Check sheet for the modelled part. Datum: model origin and axes. Units: mm. A direction names the side the tool comes from. Round coordinates to 2 decimals unless told otherwise and drop trailing zeros. Order: outer loops, then holes, each group sorted by start corner. A loop starts at its lowest first (then second) coordinate and runs counter-clockwise, first axis right, second up. Notation, with made-up numbers: (-35.75, 15.5) -> (-24.75, 15.5) arc R15 cw to (-24.75, 38.5) -> close; hole circle Ø2 at (14.5, 67). An arc over 180 degrees is marked (long way). Answer in a Markdown table with one row per item. Add a question column.
1. Sectioned sample at C-C, the plane y = 439. Record the boundary of the cut face in (x, z), then the cut area to 3 significant figures.
2. Sectioned sample at B-B, the plane y = 164. Record the boundary of the cut face in (x, z).
3. Access from +Z, -Z, +X, -X, +Y, -Y to the whole of each face (thin tool, end or side, straight path). Record for faces 1 (the flat face through (370, 93, 0)), 2 (the flat face through (0, 507, -20)), 3 (the flat face through (379, 156, -23.207)).
4. Sectioned sample at D-D, the plane x = 431. Count the separate pieces of the cut face and the enclosed holes in it, then the cut area to 3 significant figures.
5. Material ranges on L1, parallel to Y at x = 413, z = -40; L2, parallel to Y at x = 228, z = -47; L3, parallel to X at y = 914.5, z = -28.5, recorded low to high. Write a range as from..to.
6. Draft check along Y on faces 4 (the flat face through (370, 1000, -20)), 5 (the flat face through (50, 93, -30)), 6 (the flat face through (750, 507, -20)). Enter one of: +Y half, -Y half, draft (parallel to the pull), parting line (faces both ways), or undercut.
7. Depth check by flat-ended pin: P1, Ø4, axis at x = 593, z = 8.5, coming from the -Y side; P2, Ø12, axis at x = 413, z = 8.5, coming from the +Y side. Enter the tip coordinate at first touch or a pass-through.
8. Sectioned sample at A-A, the plane z = -11. Record the boundary of the cut face in (x, y).
```python
from build123d import *

# Parameters (mm, degrees)
F0_W      = 750
F0_H      = 1000
F1_DEPTH  = 20
F2_W      = 750
F2_H      = 1000
F2_W_2    = 650
F2_H_2    = 900
F3_DEPTH  = 60
F4_R      = 15
F5_W      = 650
F5_H      = 40
F6_DEPTH  = 60
F8_DEPTH  = 500
F10_DEPTH = 242


with BuildPart() as f1:
    # F0 (on Top) → F1 (new body)
    with BuildSketch(Plane.XY):
        with Locations((375, 500)):
            Rectangle(F0_W, F0_H)
    extrude(amount=F1_DEPTH)

    # F2 (on face) → F3 (join)
    with BuildSketch(Plane(origin=(0, 0, 0), x_dir=(1, 0, 0), z_dir=(0, 0, -1))):
        with Locations((375, -500)):
            Rectangle(F2_W, F2_H)
        with Locations((375, -500)):
            Rectangle(F2_W_2, F2_H_2, mode=Mode.SUBTRACT)
    extrude(amount=F3_DEPTH)

    # F4
    f4_edges = [f1.edges().sort_by_distance(p)[0] for p in [
        (750, 500, 20),
        (750, 1000, -20),
        (750, 500, -60),
        (750, 0, -20),
        (375, 0, 20),
        (375, 0, -60),
        (0, 0, -20),
        (0, 1000, -20),
        (0, 500, 20),
        (0, 500, -60),
        (375, 1000, 20),
        (375, 1000, -60),
    ]]
    fillet(f4_edges, radius=F4_R)

    # F5 (on face) → F6 (join)
    with BuildSketch(Plane(origin=(0, 0, 0), x_dir=(1, 0, 0), z_dir=(0, 0, -1))):
        with Locations((375, -155.55052)):
            Rectangle(F5_W, F5_H)
        with Locations((375, -371.085923)):
            Rectangle(F5_W, F5_H)
        with Locations((375, -586.024683)):
            Rectangle(F5_W, F5_H)
        with Locations((375, -802.115779)):
            Rectangle(F5_W, F5_H)
    extrude(amount=F6_DEPTH)

    # F7 (on face) → F8 (cut)
    with BuildSketch(Plane.XZ.offset(-351.085923)):
        with BuildLine():
            Line((678.736282, -38.204683), (678.374153, -38.204684))
            ThreePointArc((678.374153, -38.204684), (678.555218, -38.206869), (678.736282, -38.204683))
        make_face()
        with BuildLine():
            Line((71.454815, -38.206869), (678.374153, -38.204684))
            Line((678.374153, -38.204684), (678.736282, -38.204683))
            ThreePointArc((678.736282, -38.204683), (686.054644, -30.616317), (678.55519, -23.206869))
            Line((678.55519, -23.206869), (71.454761, -23.206876))
            ThreePointArc((71.454761, -23.206876), (63.954792, -30.7069), (71.454815, -38.206869))
        make_face()
    extrude(amount=-F8_DEPTH, mode=Mode.SUBTRACT)

    # F9 (on face) → F10 (cut)
    with BuildSketch(Plane.XZ.offset(-351.085923)):
        with BuildLine():
            Line((678.55519, -23.206869), (71.454788, -23.206876))
            ThreePointArc((71.454788, -23.206876), (63.954792, -30.706886), (71.454815, -38.206869))
            Line((71.454815, -38.206869), (678.374153, -38.204684))
            ThreePointArc((678.374153, -38.204684), (686.054644, -30.797395), (678.55519, -23.206869))
        make_face()
    extrude(amount=F10_DEPTH, mode=Mode.SUBTRACT)


solid = f1.part
```
Answer key:
| question | item | result |
|---|---|---|
| 1 | outline | (0, -45) arc R15 ccw to (15, -60) -> (50, -60) -> (50, 0) -> (700, 0) -> (700, -60) -> (735, -60) arc R15 ccw to (750, -45) -> (750, 5) arc R15 ccw to (735, 20) -> (15, 20) arc R15 ccw to (0, 5) -> close |
| 1 | area | 20,800 mm² |
| 2 | outline | (0, -45) arc R15 ccw to (15, -60) -> (735, -60) arc R15 ccw to (750, -45) -> (750, 5) arc R15 ccw to (735, 20) -> (15, 20) arc R15 ccw to (0, 5) -> close; hole (71.45, -38.21) -> (678.37, -38.2) arc R7.5 ccw (long way) to (678.56, -23.21) -> (71.45, -23.21) arc R7.5 ccw to start |
| 3 | face 1 | -Z |
| 3 | face 2 | +Z, -Z, -X, +Y, -Y |
| 3 | face 3 | none |
| 4 | separate pieces | 5 |
| 4 | enclosed holes | 0 |
| 4 | area | 33,000 mm² |
| 5 | L1 | y = 0..50, 135.55..175.55, 351.09..391.09, 566.02..606.02, 782.12..822.12, 950..1000 |
| 5 | L2 | y = 0.13..50, 135.55..175.55, 351.09..391.09, 566.02..606.02, 782.12..822.12, 950..999.87 |
| 5 | L3 | x = 0..50, 700..750 |
| 6 | face 4 | +Y half |
| 6 | face 5 | undercut |
| 6 | face 6 | draft |
| 7 | P1 | stops at y = 0.08 |
| 7 | P2 | stops at y = 1000 |
| 8 | outline | (0, 15) arc R15 ccw to (15, 0) -> (735, 0) arc R15 ccw to (750, 15) -> (750, 985) arc R15 ccw to (735, 1000) -> (15, 1000) arc R15 ccw to (0, 985) -> close; hole (50, 50) -> (700, 50) -> (700, 135.55) -> (50, 135.55) -> close; hole (50, 175.55) -> (700, 175.55) -> (700, 351.09) -> (50, 351.09) -> close; hole (50, 391.09) -> (700, 391.09) -> (700, 566.02) -> (50, 566.02) -> close; hole (50, 606.02) -> (700, 606.02) -> (700, 782.12) -> (50, 782.12) -> close; hole (50, 822.12) -> (700, 822.12) -> (700, 950) -> (50, 950) -> close |
